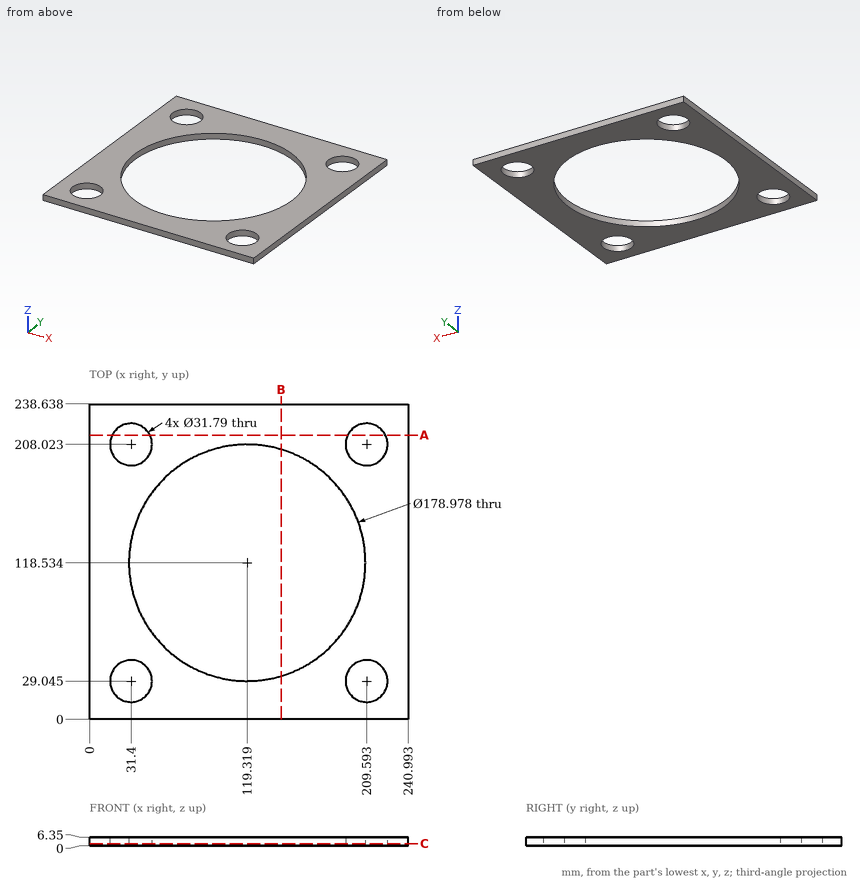
Geometry: see drawing. Coordinates: mm, zero at the bounding-box minimum. Round coordinates to 2 decimals unless told otherwise and drop trailing zeros. Order: outer loops, then holes, each group sorted by start corner. A loop starts at its lowest first (then second) coordinate and runs counter-clockwise, first axis right, second up. Notation, with made-up numbers: (86, -23) -> (131, -23) arc R28 cw to (131, 6) -> close; hole circle Ø4 at (79.25, 77.25). An arc over 180 degrees is marked (long way). Answer as CSV lines item,"result".
Item 1: Section C-C, the plane z = 1.75. Return loops of the section in (x, y) (1 decimal), plus the area to 3 significant figures.
A:
outline,"(0, 0) -> (241, 0) -> (241, 238.6) -> (0, 238.6) -> close; hole circle Ø31.8 at (31.4, 29); hole circle Ø31.8 at (31.4, 208); hole circle Ø179 at (119.3, 118.5); hole circle Ø31.8 at (209.6, 29); hole circle Ø31.8 at (209.6, 208)"
area,"29,200 mm²"
Item 2: Line query: L1, parallel to X at y = 210, z = 2.75 (1 decimal); L2, parallel to X at y = 200.5, z = 4 (1 decimal); L3, parallel to Y at x = 20.5, z = 3.5 (1 decimal). Output: solid intervals per line, ascending.
A:
L1,"0 to 15.6, 47.2 to 193.8, 225.4 to 241"
L2,"0 to 17.4, 45.4 to 83.4, 155.2 to 195.6, 223.6 to 241"
L3,"0 to 17.5, 40.6 to 196.5, 219.6 to 238.6"
Item 3: Section B-B, the plane x = 145. Return loops of the section in (y, z).
A:
outline,"(0, 0) -> (32.81, 0) -> (32.81, 6.35) -> (0, 6.35) -> close; (204.26, 0) -> (238.64, 0) -> (238.64, 6.35) -> (204.26, 6.35) -> close"
Item 4: Section A-A, the plane y = 215. Count the separate pieces of the cut face and the enclosed holes in it, plus the area to 3 significant figures.
A:
separate pieces,"3"
enclosed holes,"0"
area,"1,170 mm²"
